The listing builds one solid part. Answer for the finished solid, in the listing's coordinates (mm). Coordinates: 2 decimals unless noted, no trailing zeros. Order: outer loops, then holes, each group sorted by start corner. A loop starts at its lowest first (then second) coordinate and runs counter-clockwise, first axis right, second up. Notation, with made-up numbers: (62, 6.25) -> (76, 6.25) arc R17 cw to (76, 25.25) -> close; hole circle Ø3 at (89.5, 81). An arc over 180 degrees is marked (long way). Put each result on its own line as item: value. Start each with the question number.
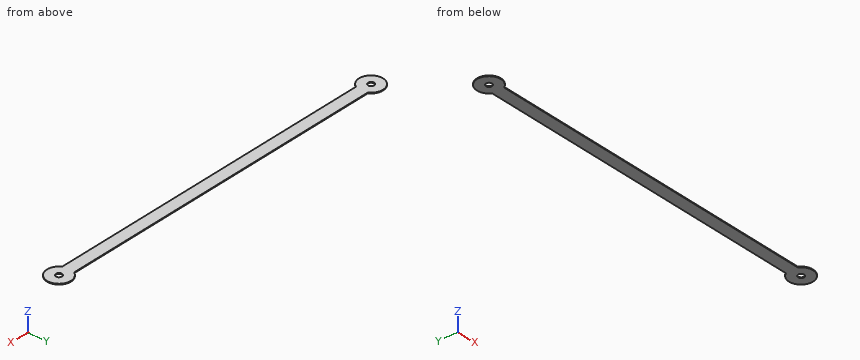
```python
from build123d import *

# Parameters (mm, degrees)
SKETCH1_R           = 1
BOSS_EXTRUDE1_DEPTH = 0.254
CUT_EXTRUDE1_DEPTH  = 1.254


with BuildPart() as part:
    # Sketch1 → Boss-Extrude1 (new body)
    with BuildSketch(Plane.XY):
        with BuildLine():
            Line((0, 4), (118, 4))
            ThreePointArc((118, 4), (122, 0), (118, -4))
            Line((118, -4), (0, -4))
            ThreePointArc((0, -4), (-4, 0), (0, 4))
        make_face()
        Circle(SKETCH1_R, mode=Mode.SUBTRACT)
        with Locations((118, 0)):
            Circle(SKETCH1_R, mode=Mode.SUBTRACT)
    extrude(amount=BOSS_EXTRUDE1_DEPTH)

    # Sketch2 → Cut-Extrude1 (cut, through all)
    with BuildSketch(Plane(origin=(0, 0, 0), x_dir=(-1, 0, 0), z_dir=(0, 0, -1))):
        with BuildLine():
            Line((-114.535898385, 2), (-3.464101615, 2))
            ThreePointArc((-3.464101615, 2), (-2, 3.464101615), (0, 4))
            Line((0, 4), (-118, 4))
            ThreePointArc((-118, 4), (-116, 3.464101615), (-114.535898385, 2))
        make_face()
        with BuildLine():
            Line((-114.535898385, -2), (-3.464101615, -2))
            ThreePointArc((-3.464101615, -2), (-2, -3.464101615), (0, -4))
            Line((0, -4), (-118, -4))
            ThreePointArc((-118, -4), (-116, -3.464101615), (-114.535898385, -2))
        make_face()
    extrude(amount=-CUT_EXTRUDE1_DEPTH, mode=Mode.SUBTRACT)


solid = part.part
```
(1) This flat-tipped pin is pushed along its axis until it touches: P1, Ø1.8, axis at x = 0, y = 0, coming from the +Z side. Where does it stop, or does it pass through?
(2) The part is cut by section A-A on z = 0.1. Determine the outline of the cut face in (x, y).
(3) Find the intervals of material crossed by L1, parallel to Y at x = 0, z = 0.2; L2, parallel to Y at x = 78, z = 0.05; L3, parallel to X at y = 0.5, z = 0.2, in increasing order.
Worked out:
1. P1: through
2. outline: (3.46, -2) -> (114.54, -2) arc R4 ccw (long way) to (114.54, 2) -> (3.46, 2) arc R4 ccw (long way) to start; hole circle Ø2 at (0, 0); hole circle Ø2 at (118, 0)
3. L1: -4 to -1, 1 to 4
3. L2: -2 to 2
3. L3: -3.97 to -0.87, 0.87 to 117.13, 118.87 to 121.97
